```python
from build123d import *

# Parameters (mm, degrees)
F0_R     = 29.21
F1_DEPTH = 0.762
F2_R     = 22.86
F3_DEPTH = 11.938


with BuildPart() as f1:
    # F0 (on Top) → F1 (new body)
    with BuildSketch(Plane.XY):
        Circle(F0_R)
    extrude(amount=F1_DEPTH)

    # F2 (on face) → F3 (join)
    with BuildSketch(Plane.XY.offset(0.762)):
        Circle(F2_R)
    extrude(amount=F3_DEPTH)

    # F4 (on Front) → F5 (revolve, cut)
    with BuildSketch(Plane.XZ):
        Polygon((0, 39.243), (0, 0), (18.8595, 0), (12.7508, 39.243), align=None)
    revolve(axis=Axis((0, 0, 19.6215), (0, 0, 1)), mode=Mode.SUBTRACT)


solid = f1.part
```
The model under review builds one solid part; all positions refer to its coordinate system, in mm. A direction names the side the tool comes from. Round coordinates to 2 decimals unless told otherwise and drop trailing zeros. Loops run counter-clockwise (first coordinate to the right, second up) from the corner with the lowest first, then second, coordinate; pieces in that order, holes last. Notation, with made-up numbers: (9.5, -21.75) -> (53.5, -21.75) arc R10 cw to (53.5, -7.75) -> close; hole circle Ø3 at (81, 13.25). An arc over 180 degrees is marked (long way). Answer as a JSON object with one key per item and string values. Group by question number.
1) For line 1 (X direction, y = -4.5, z = 1); line 2 (X direction, y = 3, z = 2.25); line 3 (Z direction, x = 7, y = -22), list the stretches that pass through material, from the lowest coordinate up. Write a range as [from, to].
2) We need section D-D on y = -22. Write out the cut boundary in (x, z).
3) We need section C-C on z = 5.75. Write out the cut boundary in (x, y).
4) Mouldability with a two-part tool opening along Y and no side actions: class faces 3 (the face through (-21.53, 19.74, 0.38)), 4 (the face through (-0.4, -19.1, 0)), 5 (the face through (16.614, 5.232, 9.261)) as released by +Y, released by -Y, zero draft, split by the parting line, or undercut.
5) For pin 1 Ø1.5 at (y, z) = (-7, 7.5) entering from +X; pin 2 Ø4 at (x, z) = (21.5, 10) entering from -Y; pin 3 Ø2 at (y, z) = (8.5, 9) entering from -X, all flat-tipped, find the tip position at first contact; note any pin that passes through.
6) We need section A-A on x = 0. Write out the cut boundary in (y, z).
7) For faces 1 (the face through (-2, -17, 12.7)), 2 (the face through (21.804, 6.867, 6.647)), list the 3-axis set-ups (+Z, -Z, +X, -X, +Y, -Y) from which the entire face can be reached by the end or side of a thin tool; tool diameter is ignored.
Result set:
{
 "1": {"line 1": "[-22.41, -18.15], [18.15, 22.41]", "line 2": "[-22.66, -18.26], [18.26, 22.66]", "line 3": "[0, 0.76]"},
 "2": {"outline": "(-19.22, 0) -> (19.22, 0) -> (19.22, 0.76) -> (6.21, 0.76) -> (6.21, 12.7) -> (-6.21, 12.7) -> (-6.21, 0.76) -> (-19.22, 0.76) -> close"},
 "3": {"outline": "circle Ø45.72 at (0, 0); hole circle Ø35.93 at (0, 0)"},
 "4": {"face 3": "split by the parting line", "face 4": "zero draft", "face 5": "undercut"},
 "5": {"pin 1": "x = 21.99", "pin 2": "y = -11.93", "pin 3": "x = -21.59"},
 "6": {"outline": "(-29.21, 0) -> (-18.86, 0) -> (-16.88, 12.7) -> (-22.86, 12.7) -> (-22.86, 0.76) -> (-29.21, 0.76) -> close; (16.88, 12.7) -> (18.86, 0) -> (29.21, 0) -> (29.21, 0.76) -> (22.86, 0.76) -> (22.86, 12.7) -> close"},
 "7": {"face 1": "+Z, +X, -X, +Y, -Y", "face 2": "+Z"}
}
